The listing builds one solid part. Answer for the finished solid, in the listing's coordinates (mm). Face numbers are marked on the shaded views. A direction names the side the tool comes from. Round coordinates to 2 decimals unless told otherwise and drop trailing zeros. Write each loop counter-clockwise with the first axis right and the second up, starting at its lowest first coordinate (ties: lowest second). Pieces come first, ordered by that corner, then holes. Notation, with made-up numbers: (-32, 30) - (7, 30) arc R23 ccw to (7, 42) - close; hole circle Ø2 at (14.25, -31.5). An arc over 180 degrees is marked (long way). Return JSON: item names as keys, results as strings. Group by question number.
(1) Section D-D, the plane y = 7.5 is taken. Write down the section's boundary in (x, z), then the cut area to 3 significant figures.
(2) Section B-B, the plane y = 4.5 is taken. Write down the section's boundary in (x, z).
(3) Find the intervals of material crossed by line 1 along X through (y, z) = (4.5, 2.75); line 2 along Y through (x, z) = (-5.25, -1); line 3 along Z through (x, y) = (0, 16.5), in increasing order. Write a range as [from, to].
(4) Section A-A, the plane z = 0 is taken. Write down the section's boundary in (x, y).
(5) Section C-C, the plane y = 15 is taken. Write down the section's boundary in (x, z), then the cut area to 3 significant figures.
(6) Each of these flat-tipped pins is pushed along its axis until it touches: pin 1 (1 mm diameter, centred on x = 4.5, y = 4, fed in from -Z); pin 2 (2 mm diameter, centred on x = -0.5, z = -5.5, fed in from +Y); pin 3 (4 mm diameter, centred on y = 3, z = -1, fed in from +X). Where does it stop, or does it pass through?
(7) Which of the six approach directions +Z, -Z, +X, -X, +Y, -Y give full straight-line access (tool end or side, diameter ignored) to the marked faces 1, 2, 3, 4 and 5?
```python
from build123d import *

# Parameters (mm, degrees)
BOSS_EXTRUDE1_DEPTH = 4.8
SKETCH2_R           = 8.5
BOSS_EXTRUDE2_DEPTH = 1
CHAMFER1_SIZE       = 0.5


with BuildPart() as part:
    # Sketch1 → Boss-Extrude1 (new body)
    with BuildSketch(Plane(origin=(0, 0, 0), x_dir=(1, 0, 0), z_dir=(0, 1, 0))):
        Polygon((0, 6.92820323), (6, 3.464101615), (6, -3.464101615), (0, -6.92820323), (-6, -3.464101615), (-6, 3.464101615), align=None)
    extrude(amount=BOSS_EXTRUDE1_DEPTH)

    # Sketch2 → Boss-Extrude2 (add)
    with BuildSketch(Plane(origin=(0, 4.8, 0), x_dir=(1, 0, 0), z_dir=(0, 1, 0))):
        with Locations(Location((0, 0, 0), (0, 0, 270))):
            Circle(SKETCH2_R)
    extrude(amount=BOSS_EXTRUDE2_DEPTH)

    # Sketch3 → Revolve1 (revolve)
    with BuildSketch(Plane.XY):
        Polygon((0, 5.8), (8.5, 5.8), (5.5, 10.996152423), (4, 10.996152423), (4, 17.996152423), (0, 17.996152423), align=None)
    revolve(axis=Axis((0, 5.8, 0), (0, 1, 0)))

    # Chamfer1
    chamfer1_edges = [part.edges().sort_by_distance(p)[0] for p in [
        (-4, 17.996152423, 0),
    ]]
    chamfer(chamfer1_edges, length=CHAMFER1_SIZE)


solid = part.part
```
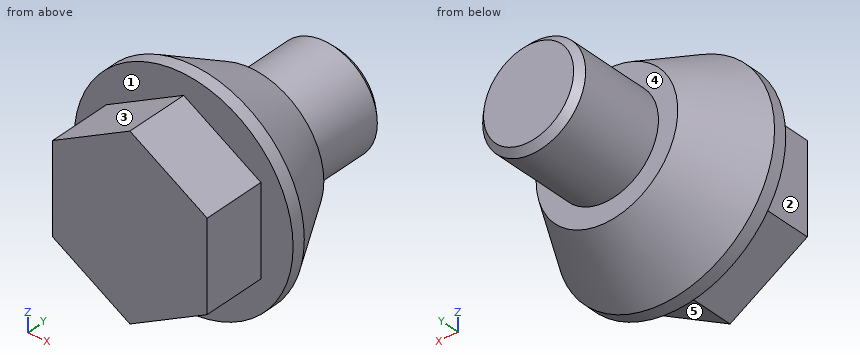
Working result:
{
 "1": {"outline": "circle Ø15.04 at (0, 0)", "area": "178 mm^2"},
 "2": {"outline": "(-6, -3.46) - (0, -6.93) - (6, -3.46) - (6, 3.46) - (0, 6.93) - (-6, 3.46) - close"},
 "3": {"line 1": "x = [-6, 6]", "line 2": "y = [0, 11]", "line 3": "z = [-4, 4]"},
 "4": {"outline": "(-8.5, 4.8) - (-6, 4.8) - (-6, 0) - (6, 0) - (6, 4.8) - (8.5, 4.8) - (8.5, 5.8) - (5.5, 11) - (4, 11) - (4, 17.5) - (3.5, 18) - (-3.5, 18) - (-4, 17.5) - (-4, 11) - (-5.5, 11) - (-8.5, 5.8) - close"},
 "5": {"outline": "circle Ø8 at (0, 0)", "area": "50.3 mm^2"},
 "6": {"pin 1": "stops at z = -4.62", "pin 2": "stops at y = 11", "pin 3": "stops at x = 8.5"},
 "7": {"face 1": "-Y", "face 2": "+Z, -Z, -X, -Y", "face 3": "+Z, -X, -Y", "face 4": "+Y", "face 5": "-Z, +X, -Y"}
}
